Verification items for the finished model (mm, model axes). Give positions to 0.01 mm unless a question says otherwise; leave off trailing zeros. Loops run counter-clockwise (first coordinate to the right, second up) from the corner with the lowest first, then second, coordinate; pieces in that order, holes last. Notation, with made-up numbers: (54, 49) -> (83, 49) arc R10 cw to (83, 60) -> close; hole circle Ø8 at (61, -12). An arc over 180 degrees is marked (long way). Answer in a Markdown table with one row per item. Add a question column.
Q1. Section check A-A on x = -37.5. Enter the section's corners in (y, z).
Q2. Section check C-C on y = 20. Enter the section's corners in (x, z), and give its area (3 significant figures).
Q3. Section check B-B on z = 11. Enter the section's corners in (x, y), and give its area (3 significant figures).
Q4. Gauge pin test, flat ends, axial feed: P1, Ø17, axis at x = 37.5, y = -30, coming from the -Z side; P2, Ø10, axis at x = 37.5, y = -30, coming from the +Z side. Record the tip position at first contact, or that the pin passes through.
Q5. Material ranges on probe 1 along Y at (x, z) = (-37.5, 17.5); probe 2 along X at (y, z) = (20, 10.5); probe 3 along X at (y, z) = (20, 18), recorded low to high.
Autodesk Inventor part; units mm, degrees
ref_plane "Work Plane3" through (37.5, -13.5, 20) normal (0, -1, 0) x (1, 0, 0)
ref_plane "YZ Plane" through (0, 0, 0) normal (1, 0, 0) x (0, 1, 0)
ref_plane "XZ Plane" through (0, 0, 0) normal (0, 1, 0) x (-1, 0, 0)
sketch "Sketch1" plane through (0, 0, 0) normal (0, 0, 1) x (1, 0, 0)
  line L0 (-52.5, -37.5) -> (52.5, -37.5)
  line L1 (52.5, -37.5) -> (52.5, 37.5)
  line L2 (52.5, 37.5) -> (-52.5, 37.5)
  line L3 (-52.5, 37.5) -> (-52.5, -37.5)
  line L4 (-52.5, -37.5) -> (52.5, 37.5) construction
  line L5 (52.5, -37.5) -> (-52.5, 37.5) construction
  point P0 (0, 0)
  dimension "d0" = 105
  dimension "d1" = 75
extrude "Extrusion1" add sketch "Sketch1" along normal blind 20
sketch "Sketch2" plane through (0, 0, 20) normal (0, 0, 1) x (1, 0, 0)
  line L0 (52.5, 37.5) -> (-52.5, 37.5)
  line L1 (-52.5, 37.5) -> (-52.5, -37.5)
  point P0 (0, 0)
  point P1 (-37.5, 20)
  point P2 (37.5, 20)
  point P3 (-37.5, -30)
  point P4 (37.5, -30)
  dimension "d4" = 75
  dimension "d5" = 17.5
  dimension "d6" = 17.5
  dimension "d7" = 15
  dimension "d8" = 50
  dimension "d9" = 50
  dimension "d10" = 75
  dimension "d11" = 15
hole "Hole1" at (-37.5, 20, 20) at (37.5, 20, 20) at (-37.5, -30, 20) at (37.5, -30, 20) direction (0, 0, -1) diameter 6.4 end through all counterbore diameter 13 counterbore depth 6.5
sketch "Sketch4" plane through (52.5, -37.5, 0) normal (1, 0, 0) x (0, 0, -1)
  line L0 (0, 75) -> (-20, 75)
  line L1 (-20, 75) -> (0, 75)
  line L2 (0, 75) -> (0, 65)
  line L3 (0, 65) -> (-20, 65)
  line L4 (-20, 65) -> (-20, 75)
  dimension "d19" = 20
  dimension "d20" = 10
extrude "Extrusion2" cut sketch "Sketch4" against normal through all
sketch "Sketch5" plane through (-52.5, -37.5, 0) normal (0, -1, 0) x (1, 0, 0)
  point P0 (52.5, 0)
sketch "Sketch7" plane through (0, 0, 20) normal (0, 0, 1) x (1, 0, 0)
  line L0 (37.5265, 13.5317) -> (37.5265, -23.5001)
  circle A0 centre (37.5, -30) radius 6.5
  line L1 (37.5265, -23.5001) -> (37.5265, -13.5001)
  line L2 (37.5265, -13.5001) -> (40.9265, -13.5001)
  line L3 (40.9265, -13.5001) -> (34.1265, -13.5001)
  line L4 (37.5265, -13.5001) -> (39.2265, -13.5001)
  line L5 (39.2265, -13.5001) -> (35.8265, -13.5001)
  point P0 (0, 0)
  dimension "d41" = 10
  dimension "d42" = 3.4
  dimension "d43" = 6.8
  dimension "d44" = 1.7
  dimension "d45" = 3.4
sketch "Sketch8" plane through (0, 0, 20) normal (0, 0, 1) x (1, 0, 0)
  circle A0 centre (37.5, -30) radius 6.5
  line L0 (37.5, -23.5) -> (37.5, -13.5)
  point P0 (0, 0)
  dimension "d25" = 10
ref_plane "Work Plane3" through (37.5, -13.5, 20) normal (0, -1, 0) x (1, 0, 0)
ref_plane "Work Plane4" through (37.5265, -13.5001, 20) normal (0, -1, 0) x (1, 0, 0)
sketch "Sketch10" plane through (37.5265, -13.5001, 20) normal (0, -1, 0) x (1, 0, 0)
  line L0 (1.6997, -0.0003) -> (1.6997, 1.6997)
  line L1 (-1.7001, -0.0003) -> (-1.7001, 1.6997)
  point P0 (-37.5265, -20)
  dimension "d46" = 1.7
  dimension "d47" = 1.7
hole "Hole3" at (35.8265, -13.5001, 21.6997) direction (0, 1, 0) diameter 3 depth 17
sketch "Sketch12" plane through (37.5265, -13.5001, 20) normal (0, -1, 0) x (1, 0, 0)
  line L0 (1.6597, 0) -> (1.7401, 0)
  line L1 (1.6999, 0) -> (1.6999, 1.7)
  point P0 (-37.5265, -20)
  dimension "d59" = 1.7
properties part number "Soporte"
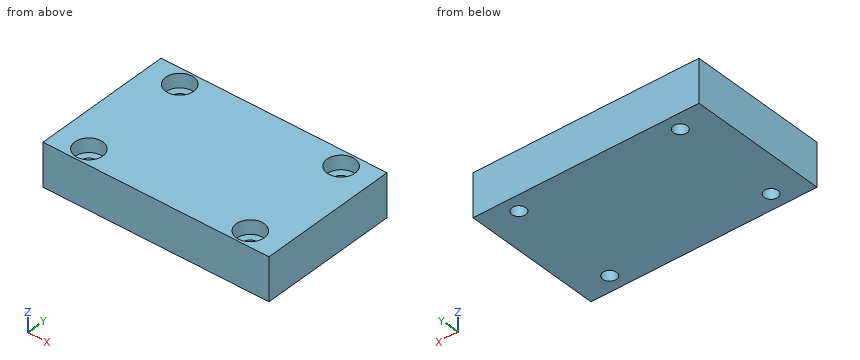
Taken from the geometry:
| question | item | result |
|---|---|---|
| 1 | outline | (-37.5, 0) -> (-33.2, 0) -> (-33.2, 13.5) -> (-36.5, 13.5) -> (-36.5, 20) -> (-37.5, 20) -> close; (-26.8, 0) -> (16.8, 0) -> (16.8, 13.5) -> (13.5, 13.5) -> (13.5, 20) -> (-23.5, 20) -> (-23.5, 13.5) -> (-26.8, 13.5) -> close; (23.2, 0) -> (27.5, 0) -> (27.5, 20) -> (26.5, 20) -> (26.5, 13.5) -> (23.2, 13.5) -> close |
| 2 | outline | (-52.5, 0) -> (-40.7, 0) -> (-40.7, 13.5) -> (-44, 13.5) -> (-44, 20) -> (-52.5, 20) -> close; (-34.3, 0) -> (34.3, 0) -> (34.3, 13.5) -> (31, 13.5) -> (31, 20) -> (-31, 20) -> (-31, 13.5) -> (-34.3, 13.5) -> close; (40.7, 0) -> (52.5, 0) -> (52.5, 20) -> (44, 20) -> (44, 13.5) -> (40.7, 13.5) -> close |
| 2 | area | 1,760 mm² |
| 3 | outline | (-52.5, -37.5) -> (52.5, -37.5) -> (52.5, 27.5) -> (-52.5, 27.5) -> close; hole circle Ø6.4 at (-37.5, -30); hole circle Ø6.4 at (-37.5, 20); hole circle Ø6.4 at (37.5, -30); hole circle Ø6.4 at (37.5, 20) |
| 3 | area | 6,700 mm² |
| 4 | P1 | stops at z = 0 |
| 4 | P2 | stops at z = 13.5 |
| 5 | probe 1 | y = -37.5 to -36.5, -23.5 to 13.5, 26.5 to 27.5 |
| 5 | probe 2 | x = -52.5 to -40.7, -34.3 to 34.3, 40.7 to 52.5 |
| 5 | probe 3 | x = -52.5 to -44, -31 to 31, 44 to 52.5 |
